Design review of the part built by this model. Coordinates are the model's own, in mm. A direction names the side the tool comes from. Round coordinates to 2 decimals unless told otherwise and drop trailing zeros. Loops run counter-clockwise (first coordinate to the right, second up) from the corner with the lowest first, then second, coordinate; pieces in that order, holes last. Notation, with made-up numbers: M 42.25,40 L 88.25,40 A28 ccw 88.25,70 Z; hole C 34,15 d10. An arc over 180 degrees is marked long. Use a Markdown table: item, result.
from build123d import *

# Parameters (mm, degrees)
SKETCH1_W           = 50
SKETCH1_H           = 23
BOSS_EXTRUDE1_DEPTH = 2
SKETCH2_W           = 50
SKETCH2_H           = 23
BOSS_EXTRUDE2_DEPTH = 6
SKETCH3_W           = 46
SKETCH3_H           = 20
CUT_EXTRUDE1_DEPTH  = 4
SKETCH4_W           = 46
SKETCH4_H           = 4
CUT_EXTRUDE2_DEPTH  = 4
SKETCH5_W           = 46
SKETCH5_H           = 21.5
CUT_EXTRUDE3_DEPTH  = 2
SKETCH6_W           = 2
SKETCH6_H           = 21.5
BOSS_EXTRUDE3_DEPTH = 2
SKETCH7_W           = 2
SKETCH7_H           = 21.5
BOSS_EXTRUDE4_DEPTH = 2
SKETCH8_W           = 15
SKETCH8_H           = 6
CUT_EXTRUDE5_DEPTH  = 2


with BuildPart() as part:
    # Sketch1 → Boss-Extrude1 (new body)
    with BuildSketch(Plane.XY):
        Rectangle(SKETCH1_W, SKETCH1_H)
    extrude(amount=BOSS_EXTRUDE1_DEPTH)

    # Sketch2 → Boss-Extrude2 (add)
    with BuildSketch(Plane.XY.offset(2)):
        Rectangle(SKETCH2_W, SKETCH2_H)
    extrude(amount=BOSS_EXTRUDE2_DEPTH)

    # Sketch3 → Cut-Extrude1 (cut)
    with BuildSketch(Plane.XY.offset(8)):
        Rectangle(SKETCH3_W, SKETCH3_H)
    extrude(amount=-CUT_EXTRUDE1_DEPTH, mode=Mode.SUBTRACT)

    # Sketch4 → Cut-Extrude2 (cut)
    with BuildSketch(Plane.XZ.offset(-10)):
        with Locations((0, 6)):
            Rectangle(SKETCH4_W, SKETCH4_H)
    extrude(amount=-CUT_EXTRUDE2_DEPTH, mode=Mode.SUBTRACT)

    # Sketch5 → Cut-Extrude3 (cut)
    with BuildSketch(Plane.XY.offset(4)):
        with Locations((0, 0.75)):
            Rectangle(SKETCH5_W, SKETCH5_H)
    extrude(amount=-CUT_EXTRUDE3_DEPTH, mode=Mode.SUBTRACT)

    # Sketch6 → Boss-Extrude3 (add)
    with BuildSketch(Plane.ZY.offset(-23)):
        with Locations((7, 0.75)):
            Rectangle(SKETCH6_W, SKETCH6_H)
    extrude(amount=BOSS_EXTRUDE3_DEPTH)

    # Sketch7 → Boss-Extrude4 (add)
    with BuildSketch(Plane(origin=(-23, 0, 0), x_dir=(0, 0, -1), z_dir=(1, 0, 0))):
        with Locations((-7, 0.75)):
            Rectangle(SKETCH7_W, SKETCH7_H)
    extrude(amount=BOSS_EXTRUDE4_DEPTH)

    # Sketch8 → Cut-Extrude5 (cut)
    with BuildSketch(Plane.XY.offset(2)):
        with Locations((0, 11.5)):
            Rectangle(SKETCH8_W, SKETCH8_H)
    extrude(amount=-CUT_EXTRUDE5_DEPTH, mode=Mode.SUBTRACT)


solid = part.part
1. Take a section at D-D on x = -18. Give the boundary of the cut face in (y, z).
Check values:
| item | result |
|---|---|
| outline | M -11.5,0 L 11.5,0 L 11.5,2 L -10,2 L -10,8 L -11.5,8 Z |
2. Machinability: for faces 1 (the face through (-21, 1, 7)), 2 (the face through (23, 1, 4)), 3 (the face through (-7.5, 10, 1)), which of the approach directions +Z, -Z, +X, -X, +Y, -Y give a long, thin tool a straight path to every point of the face, cutting with its end or side? Answer none if there is none.
Check values:
| item | result |
|---|---|
| face 1 | +Z, +Y |
| face 2 | +Y |
| face 3 | +Z, -Z, +Y |
3. Wall thickness on line 1 along X through (y, z) = (-5.25, 3); line 2 along X through (y, z) = (9.5, 1.5); line 3 along Z through (x, y) = (22.5, 5): over which ranges is each line inside the solid? List them lowest first. Write a range as from..to.
Check values:
| item | result |
|---|---|
| line 1 | x = -25..-23, 23..25 |
| line 2 | x = -25..-7.5, 7.5..25 |
| line 3 | z = 0..2, 6..8 |
4. Take a section at B-B on z = 4.75. Give the boundary of the cut face in (x, y).
Check values:
| item | result |
|---|---|
| outline | M -25,-11.5 L 25,-11.5 L 25,11.5 L 23,11.5 L 23,-10 L -23,-10 L -23,11.5 L -25,11.5 Z |
5. Insertion check: pin 1 (0.6 mm diameter, centred on x = 22.5, y = 2.5, fed in from -Z); pin 2 (10 mm diameter, centred on x = 2.5, y = 5.5, fed in from +Z); pin 3 (2 mm diameter, centred on x = 1, z = 0.5, fed in from +Y). Each pin has a flat end and moves straight along its axis. Give the tip position at first contact, or say it passes through.
Check values:
| item | result |
|---|---|
| pin 1 | stops at z = 0 |
| pin 2 | stops at z = 2 |
| pin 3 | stops at y = 8.5 |
6. Take a section at A-A on x = 22. Give the boundary of the cut face in (y, z).
Check values:
| item | result |
|---|---|
| outline | M -11.5,0 L 11.5,0 L 11.5,2 L -10,2 L -10,6 L 11.5,6 L 11.5,8 L -11.5,8 Z |
7. The part is to be moulded in two halves that separate along X. For faces 4 (the face through (25, 0, 4)), 5 (the face through (21, 1, 7)), 6 (the face through (-17.6, 11.5, 1.6)), 7 (the face through (7.5, 10, 1)), say which applies: pulls with the +X half, pulls with the -X half, needs draft (parallel to the pull), parting line crosses it, or undercut.
Check values:
| item | result |
|---|---|
| face 4 | pulls with the +X half |
| face 5 | undercut |
| face 6 | needs draft |
| face 7 | undercut |
8. Take a section at C-C on y = 4. Give the boundary of the cut face in (x, z), and give its area (3 significant figures).
Check values:
| item | result |
|---|---|
| outline | M -25,0 L 25,0 L 25,8 L 21,8 L 21,6 L 23,6 L 23,2 L -23,2 L -23,6 L -21,6 L -21,8 L -25,8 Z |
| area | 132 mm² |
